The model under review builds one solid part; all positions refer to its coordinate system, in mm. Round coordinates to 2 decimals unless told otherwise and drop trailing zeros. Write each loop counter-clockwise with the first axis right and the second up, starting at its lowest first coordinate (ties: lowest second). Pieces come first, ordered by that corner, then holes. Notation, with made-up numbers: (-10.75, 46.5) - (7.25, 46.5) arc R24 ccw to (7.25, 57.5) - close; hole circle Ø8 at (-40, 8.5). An arc over 180 degrees is marked (long way). Write each question's results on one line, items separated by ' | '.
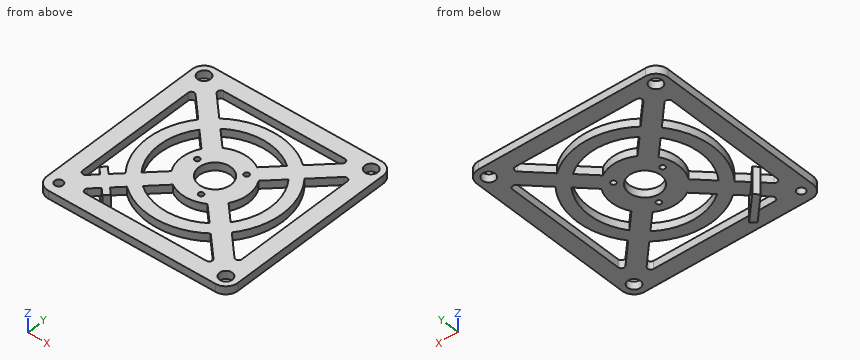
```python
from build123d import *

# Parameters (mm, degrees)
SKETCH1_R                  = 4
SKETCH1_R_2                = 10
EXTRUDE1_DEPTH             = 2.5
FILLET1_R                  = 2
EXTRUDE5_REACH             = 87
SKETCH6_R                  = 1.6
EXTRUDE6_START             = -5
SKETCH7_R                  = 4
EXTRUDE6_DEPTH             = 5
SKETCH10_R                 = 2.6
EXTRUDE7_DEPTH             = 10
EXTRUDE8_DEPTH             = 12
EXTRUDE8_DIRECTION_2_REACH = 87
SKETCH12_R                 = 1.3
EXTRUDE9_DEPTH             = 10


with BuildPart() as part:
    # Sketch1 → Extrude1 (new, symmetric)
    with BuildSketch(Plane.XY):
        with BuildLine():
            Line((52.5, 60), (-52.5, 60))
            ThreePointArc((-52.5, 60), (-57.803300859, 57.803300859), (-60, 52.5))
            Line((-60, 52.5), (-60, -52.5))
            ThreePointArc((-60, -52.5), (-57.803300859, -57.803300859), (-52.5, -60))
            Line((-52.5, -60), (52.5, -60))
            ThreePointArc((52.5, -60), (57.803300859, -57.803300859), (60, -52.5))
            Line((60, -52.5), (60, 52.5))
            ThreePointArc((60, 52.5), (57.803300859, 57.803300859), (52.5, 60))
        make_face()
        with BuildLine():
            Line((-50, 42.928932188), (-33.378874872, 26.30780706))
            ThreePointArc((-33.378874872, 26.30780706), (-42.5, 0), (-33.378874872, -26.30780706))
            Line((-33.378874872, -26.30780706), (-50, -42.928932188))
            Line((-50, -42.928932188), (-50, 42.928932188))
        make_face(mode=Mode.SUBTRACT)
        with Locations((-52.5, -52.5)):
            Circle(SKETCH1_R, mode=Mode.SUBTRACT)
        with BuildLine():
            Line((-42.928932188, -50), (-26.30780706, -33.378874872))
            ThreePointArc((-26.30780706, -33.378874872), (0, -42.5), (26.30780706, -33.378874872))
            Line((26.30780706, -33.378874872), (42.928932188, -50))
            Line((42.928932188, -50), (-42.928932188, -50))
        make_face(mode=Mode.SUBTRACT)
        with Locations((52.5, -52.5)):
            Circle(SKETCH1_R, mode=Mode.SUBTRACT)
        with BuildLine():
            Line((50, -42.928932188), (33.378874872, -26.30780706))
            ThreePointArc((33.378874872, -26.30780706), (42.5, 0), (33.378874872, 26.30780706))
            Line((33.378874872, 26.30780706), (50, 42.928932188))
            Line((50, 42.928932188), (50, -42.928932188))
        make_face(mode=Mode.SUBTRACT)
        with Locations((52.5, 52.5)):
            Circle(SKETCH1_R, mode=Mode.SUBTRACT)
        with BuildLine():
            Line((42.928932188, 50), (26.30780706, 33.378874872))
            ThreePointArc((26.30780706, 33.378874872), (0, 42.5), (-26.30780706, 33.378874872))
            Line((-26.30780706, 33.378874872), (-42.928932188, 50))
            Line((-42.928932188, 50), (42.928932188, 50))
        make_face(mode=Mode.SUBTRACT)
        with Locations((-52.5, 52.5)):
            Circle(SKETCH1_R, mode=Mode.SUBTRACT)
        with BuildLine():
            Line((-20.959363522, -28.030431334), (-10.886671196, -17.957739008))
            ThreePointArc((-10.886671196, -17.957739008), (0, -21), (10.886671196, -17.957739008))
            Line((10.886671196, -17.957739008), (20.959363522, -28.030431334))
            ThreePointArc((20.959363522, -28.030431334), (0, -35), (-20.959363522, -28.030431334))
        make_face(mode=Mode.SUBTRACT)
        with BuildLine():
            ThreePointArc((17.957739008, -10.886671196), (21, 0), (17.957739008, 10.886671196))
            Line((17.957739008, 10.886671196), (28.030431334, 20.959363522))
            ThreePointArc((28.030431334, 20.959363522), (35, 0), (28.030431334, -20.959363522))
            Line((28.030431334, -20.959363522), (17.957739008, -10.886671196))
        make_face(mode=Mode.SUBTRACT)
        with BuildLine():
            ThreePointArc((10.886671196, 17.957739008), (0, 21), (-10.886671196, 17.957739008))
            Line((-10.886671196, 17.957739008), (-20.959363522, 28.030431334))
            ThreePointArc((-20.959363522, 28.030431334), (0, 35), (20.959363522, 28.030431334))
            Line((20.959363522, 28.030431334), (10.886671196, 17.957739008))
        make_face(mode=Mode.SUBTRACT)
        with BuildLine():
            Line((-17.957739008, -10.886671196), (-28.030431334, -20.959363522))
            ThreePointArc((-28.030431334, -20.959363522), (-35, 0), (-28.030431334, 20.959363522))
            Line((-28.030431334, 20.959363522), (-17.957739008, 10.886671196))
            ThreePointArc((-17.957739008, 10.886671196), (-21, 0), (-17.957739008, -10.886671196))
        make_face(mode=Mode.SUBTRACT)
        Circle(SKETCH1_R_2, mode=Mode.SUBTRACT)
    extrude(amount=EXTRUDE1_DEPTH, both=True)

    # Fillet1
    fillet1_edges = [part.edges().sort_by_distance(p)[0] for p in [
        (50, 42.928932188, 0),
        (50, -42.928932188, 0),
        (42.928932188, 50, 0),
        (-42.928932188, 50, 0),
        (-50, 42.928932188, 0),
        (-50, -42.928932188, 0),
        (-42.928932188, -50, 0),
        (42.928932188, -50, 0),
    ]]
    fillet(fillet1_edges, radius=FILLET1_R)

    # Sketch6 → Extrude5 (cut, up to next)
    with BuildSketch(Plane(origin=(0, 0, -2.5), x_dir=(-1, 0, 0), z_dir=(0, 0, -1)), mode=Mode.PRIVATE) as extrude5_sk1:
        with Locations((-10.606601718, 10.606601718)):
            Circle(SKETCH6_R)
    extrude5_tool1 = extrude(extrude5_sk1.sketch, amount=-EXTRUDE5_REACH, mode=Mode.PRIVATE) & part.part
    # Sketch6 → Extrude5 (cut, up to next)
    with BuildSketch(Plane(origin=(0, 0, -2.5), x_dir=(-1, 0, 0), z_dir=(0, 0, -1)), mode=Mode.PRIVATE) as extrude5_sk2:
        with Locations((14.488887394, 3.882285677)):
            Circle(SKETCH6_R)
    extrude5_tool2 = extrude(extrude5_sk2.sketch, amount=-EXTRUDE5_REACH, mode=Mode.PRIVATE) & part.part
    # Sketch6 → Extrude5 (cut, up to next)
    with BuildSketch(Plane(origin=(0, 0, -2.5), x_dir=(-1, 0, 0), z_dir=(0, 0, -1)), mode=Mode.PRIVATE) as extrude5_sk3:
        with Locations((-3.882285677, -14.488887394)):
            Circle(SKETCH6_R)
    extrude5_tool3 = extrude(extrude5_sk3.sketch, amount=-EXTRUDE5_REACH, mode=Mode.PRIVATE) & part.part
    add(extrude5_tool1.solids().sort_by_distance((10.606602, 10.606602, -2.5))[0], mode=Mode.SUBTRACT)
    add(extrude5_tool2.solids().sort_by_distance((-14.488887, 3.882286, -2.5))[0], mode=Mode.SUBTRACT)
    add(extrude5_tool3.solids().sort_by_distance((3.882286, -14.488887, -2.5))[0], mode=Mode.SUBTRACT)

    # Sketch7 → Extrude6 (add)
    with BuildSketch(Plane.XY.offset(2.5).offset(EXTRUDE6_START)):
        with Locations((-52.5, -52.5)):
            Circle(SKETCH7_R)
    extrude(amount=EXTRUDE6_DEPTH)

    # Sketch10 → Extrude7 (cut)
    with BuildSketch(Plane(origin=(0, 0, -2.5), x_dir=(-1, 0, 0), z_dir=(0, 0, -1))):
        with Locations((52.5, -52.5)):
            Circle(SKETCH10_R)
    extrude(amount=-EXTRUDE7_DEPTH, mode=Mode.SUBTRACT)

    # Sketch11 → Extrude8 (add)
    with BuildSketch(Plane(origin=(0, 0, -2.5), x_dir=(-1, 0, 0), z_dir=(0, 0, -1))):
        Polygon((28.104816049, -42.954058454), (42.954058454, -28.104816049), (45.782485579, -30.933243174), (30.933243174, -45.782485579), align=None)
    extrude(amount=EXTRUDE8_DEPTH)

    # Extrude8 direction 2: up to this face of the body (flat: up to its plane)
    extrude8_direction_2_end = Plane(part.part.faces().sort_by_distance((0, 58.302943725, 2.5))[0])
    # Sketch11 → Extrude8 direction 2 (add, up to the picked face)
    with BuildSketch(Plane(origin=(0, 0, -2.5), x_dir=(-1, 0, 0), z_dir=(0, 0, -1)), mode=Mode.PRIVATE) as extrude8_direction_2_sk1:
        Polygon((28.104816049, -42.954058454), (42.954058454, -28.104816049), (45.782485579, -30.933243174), (30.933243174, -45.782485579), align=None)
    extrude8_direction_2_tool1 = split(extrude(extrude8_direction_2_sk1.sketch, amount=-EXTRUDE8_DIRECTION_2_REACH, mode=Mode.PRIVATE), bisect_by=extrude8_direction_2_end, keep=Keep.BOTH, mode=Mode.PRIVATE)
    add(extrude8_direction_2_tool1.solids().sort_by(Axis((-36.943651, -36.943651, -2.5), (0, 0, 1)))[0])

    # Sketch12 → Extrude9 (cut)
    with BuildSketch(Plane(origin=(-35.529437252, -35.529437252, 0), x_dir=(0, 0, -1), z_dir=(0.7071067811865501, 0.7071067811865449, 0))):
        with Locations(Location((5, -8.25, 0), (0, 0, 90))):
            Circle(SKETCH12_R)
        with Locations(Location((5, 8.25, 0), (0, 0, 90))):
            Circle(SKETCH12_R)
    extrude(amount=-EXTRUDE9_DEPTH, mode=Mode.SUBTRACT)


solid = part.part
```
Q1. Insertion check: P1, Ø2, axis at x = 43.5, y = 38.5, coming from the -Z side; P2, Ø6, axis at y = 1.5, z = -6, coming from the -X side. Each pin has a flat end and moves straight along its axis. Give the tip position at first contact, or say it passes through.
Evaluation:
P1: stops at z = -2.5 | P2: passes through
Q2. For probe 1 along Y at (x, z) = (0, 1); probe 2 along Y at (x, z) = (-25.5, 1.5); probe 3 along Y at (x, z) = (-27.5, 2.25), list the stretches that pass through material, from the lowest coordinate up.
Evaluation:
probe 1: y = -60 to -50, -42.5 to -35, -21 to -10, 10 to 21, 35 to 42.5, 50 to 60 | probe 2: y = -60 to -50, -34 to -18.43, 18.43 to 34, 50 to 60 | probe 3: y = -60 to -50, -34.57 to -20.43, 20.43 to 34.57, 50 to 60
Q3. We need section D-D (y = 31). State the section outline as (x, z) points.
Evaluation:
outline: (-60, -2.5) - (-50, -2.5) - (-50, 2.5) - (-60, 2.5) - close; (-38.07, -2.5) - (-16.25, -2.5) - (-16.25, 2.5) - (-38.07, 2.5) - close; (16.25, -2.5) - (38.07, -2.5) - (38.07, 2.5) - (16.25, 2.5) - close; (50, -2.5) - (60, -2.5) - (60, 2.5) - (50, 2.5) - close
Q4. We need section C-C (y = 44). State the section outline as (x, z) points.
Evaluation:
outline: (-60, -2.5) - (-36.93, -2.5) - (-36.93, 2.5) - (-60, 2.5) - close; (36.93, -2.5) - (60, -2.5) - (60, 2.5) - (36.93, 2.5) - close
Q5. We need section A-A (y = 0). State the section outline as (x, z) points.
Evaluation:
outline: (-60, -2.5) - (-50, -2.5) - (-50, 2.5) - (-60, 2.5) - close; (-42.5, -2.5) - (-35, -2.5) - (-35, 2.5) - (-42.5, 2.5) - close; (-21, -2.5) - (-10, -2.5) - (-10, 2.5) - (-21, 2.5) - close; (10, -2.5) - (21, -2.5) - (21, 2.5) - (10, 2.5) - close; (35, -2.5) - (42.5, -2.5) - (42.5, 2.5) - (35, 2.5) - close; (50, -2.5) - (60, -2.5) - (60, 2.5) - (50, 2.5) - close
